from build123d import *

# Parameters (mm, degrees)
SKETCH_1_W              = 85
SKETCH_1_H              = 40
EXTRUDE_1_DEPTH         = 4
SKETCH_2_R              = 1.51
CUT_EXTRUDE_1_DEPTH     = 10
SKETCH_3_R              = 1.51
CUT_EXTRUDE_2_DEPTH     = 10
SKETCH_5_R              = 1.51
CUT_EXTRUDE_4_DEPTH     = 10
SKETCH_6_W              = 85
SKETCH_6_H              = 25
EXTRUDE_2_DEPTH         = 4
SKETCH_7_R              = 1.51
CUT_EXTRUDE_5_DEPTH     = 3
CUT_EXTRUDE_START       = -3
SKETCH_8_R              = 1.51
CUT_EXTRUDE_6_DEPTH     = 3
CUT_EXTRUDE_7_DEPTH     = 10
SKETCH_10_R             = 1.5
CUT_EXTRUDE_8_DEPTH     = 10
SKETCH_12_OUTSIDE_W     = 108.416
SKETCH_12_OUTSIDE_H     = 88.416
CUT_EXTRUDE_9_DEPTH     = 10
SKETCH_13_W             = 85
SKETCH_13_H             = 20
CUT_EXTRUDE_10_DEPTH    = 10
FILLET_2_R              = 4
MOVE_FACE_1_DEPTH       = 4
MOVE_FACE_2_OUTLINE_R   = 1.51
MOVE_FACE_2_DEPTH       = 4
MOVE_FACE_2_2_OUTLINE_R = 1.51
MOVE_FACE_2_2_DEPTH     = 4
MOVE_FACE_3_OUTLINE_R   = 1.51
MOVE_FACE_3_DEPTH       = 4
MOVE_FACE_3_2_OUTLINE_R = 1.51
MOVE_FACE_3_2_DEPTH     = 4
CUT_EXTRUDE_11_DEPTH    = 10
FILLET_3_R              = 2
CUT_EXTRUDE_12_DEPTH    = 10
FILLET_4_R              = 2


# Read off the part's stored shape, not the designer's step: 移动面1, 移动面2, 移动面3
with BuildPart() as part:
    # 草图1 → 凸台-拉伸1 (new body)
    with BuildSketch(Plane(origin=(0, 0, 0), x_dir=(0, 0, -1), z_dir=(1, 0, 0))):
        Rectangle(SKETCH_1_W, SKETCH_1_H)
    extrude(amount=EXTRUDE_1_DEPTH)

    # 草图2 → 切除-拉伸1 (cut)
    with BuildSketch(Plane.ZY):
        with Locations((-37.5, -11)):
            Circle(SKETCH_2_R)
        with Locations((37.5, -11)):
            Circle(SKETCH_2_R)
        with Locations((37.5, 11)):
            Circle(SKETCH_2_R)
        with Locations((-37.5, 11)):
            Circle(SKETCH_2_R)
    extrude(amount=-CUT_EXTRUDE_1_DEPTH, mode=Mode.SUBTRACT)

    # 草图3 → 切除-拉伸2 (cut)
    with BuildSketch(Plane.ZY):
        with Locations((-2.5, 0)):
            Circle(SKETCH_3_R)
        with Locations((-22.5, 0)):
            Circle(SKETCH_3_R)
    extrude(amount=-CUT_EXTRUDE_2_DEPTH, mode=Mode.SUBTRACT)

    # 草图5 → 切除-拉伸4 (cut)
    with BuildSketch(Plane.ZY):
        with BuildLine():
            Line((29.5, 6), (29.5, 20))
            Line((29.5, 20), (-12.5, 20))
            Line((-12.5, 20), (-12.5, 6))
            ThreePointArc((-12.5, 6), (-9.571067812, -1.071067812), (-2.5, -4))
            Line((-2.5, -4), (19.5, -4))
            ThreePointArc((19.5, -4), (26.571067812, -1.071067812), (29.5, 6))
        make_face()
        with Locations((-2.5, 0)):
            Circle(SKETCH_5_R, mode=Mode.SUBTRACT)
    extrude(amount=-CUT_EXTRUDE_4_DEPTH, mode=Mode.SUBTRACT)

    # 草图6 → 凸台-拉伸2 (add)
    with BuildSketch(Plane.ZY):
        with Locations((0, -32.5)):
            Rectangle(SKETCH_6_W, SKETCH_6_H)
    extrude(amount=-EXTRUDE_2_DEPTH)

    # 草图7 → 切除-拉伸5 (cut)
    with BuildSketch(Plane(origin=(4, 0, 0), x_dir=(0, 0, -1), z_dir=(1, 0, 0))):
        with Locations((-10, -11)):
            Circle(SKETCH_7_R)
        with Locations((10, -11)):
            Circle(SKETCH_7_R)
    extrude(amount=-CUT_EXTRUDE_5_DEPTH, mode=Mode.SUBTRACT)

    # 草图8 → 切除-拉伸6 (cut)
    with BuildSketch(Plane.ZY.offset(CUT_EXTRUDE_START)):
        with Locations(Location((-10, -11, 0), (0, 0, 180))):
            Circle(SKETCH_8_R)
        with Locations(Location((10, -11, 0), (0, 0, 180))):
            Circle(SKETCH_8_R)
    extrude(amount=CUT_EXTRUDE_6_DEPTH, mode=Mode.SUBTRACT)

    # 草图9 → 切除-拉伸7 (cut)
    with BuildSketch(Plane(origin=(4, 0, 0), x_dir=(0, 0, -1), z_dir=(1, 0, 0))):
        Polygon((26, -14), (17.872575328, -14), (-2.448990482, -14), (-16, -14), (-16, -18), (-14, -18), (24, -18), (26, -18), align=None)
    extrude(amount=-CUT_EXTRUDE_7_DEPTH, mode=Mode.SUBTRACT)

    # 草图10 → 切除-拉伸8 (cut)
    with BuildSketch(Plane(origin=(4, 0, 0), x_dir=(0, 0, -1), z_dir=(1, 0, 0))):
        with Locations((24.52, -18.02)):
            Circle(SKETCH_10_R)
        with Locations((-14.52, -18.02)):
            Circle(SKETCH_10_R)
        with Locations((-14.52, -13.98)):
            Circle(SKETCH_10_R)
        with Locations((24.52, -13.98)):
            Circle(SKETCH_10_R)
        Polygon((26.02, -13.98), (17.872575328, -13.98), (-2.448990482, -13.98), (-16.02, -13.98), (-16.02, -18.02), (-14, -18.02), (24, -18.02), (26.02, -18.02), align=None)
    extrude(amount=-CUT_EXTRUDE_8_DEPTH, mode=Mode.SUBTRACT)

    # 草图12 outside → 切除-拉伸9 (cut)
    with BuildSketch(Plane.ZY):
        with Locations((0, -12.5)):
            Rectangle(SKETCH_12_OUTSIDE_W, SKETCH_12_OUTSIDE_H)
        with BuildLine():
            Line((-12.5, 6), (-12.5, 16))
            ThreePointArc((-12.5, 16), (-13.671572875, 18.828427125), (-16.5, 20))
            Line((-16.5, 20), (-38.5, 20))
            ThreePointArc((-38.5, 20), (-41.328427125, 18.828427125), (-42.5, 16))
            Line((-42.5, 16), (-42.5, -45))
            Line((-42.5, -45), (42.5, -45))
            Line((42.5, -45), (42.5, 16))
            ThreePointArc((42.5, 16), (41.328427125, 18.828427125), (38.5, 20))
            Line((38.5, 20), (33.5, 20))
            ThreePointArc((33.5, 20), (30.671572875, 18.828427125), (29.5, 16))
            Line((29.5, 16), (29.5, 6))
            ThreePointArc((29.5, 6), (26.571067812, -1.071067812), (19.5, -4))
            Line((19.5, -4), (-2.5, -4))
            ThreePointArc((-2.5, -4), (-9.571067812, -1.071067812), (-12.5, 6))
        make_face(mode=Mode.SUBTRACT)
    extrude(amount=-CUT_EXTRUDE_9_DEPTH, mode=Mode.SUBTRACT)

    # 草图13 → 切除-拉伸10 (cut)
    with BuildSketch(Plane.ZY):
        with Locations((0, -35)):
            Rectangle(SKETCH_13_W, SKETCH_13_H)
    extrude(amount=-CUT_EXTRUDE_10_DEPTH, mode=Mode.SUBTRACT)

    # 圆角2
    fillet_2_edges = [part.edges().sort_by_distance(p)[0] for p in [
        (2, -25, 42.5),
        (2, -25, -42.5),
    ]]
    fillet(fillet_2_edges, radius=FILLET_2_R)

    # Move Face 1 outline → Move Face 1 (add)
    with BuildSketch(Plane.YZ):
        with BuildLine():
            Line((20, 38.5), (20, 45.5))
            ThreePointArc((20, 45.5), (18.828427125, 48.328427125), (16, 49.5))
            Line((16, 49.5), (-21, 49.5))
            ThreePointArc((-21, 49.5), (-23.828427125, 48.328427125), (-25, 45.5))
            Line((-25, 45.5), (-25, 38.5))
            ThreePointArc((-25, 38.5), (-23.828427125, 41.328427125), (-21, 42.5))
            Line((-21, 42.5), (16, 42.5))
            ThreePointArc((16, 42.5), (18.828427125, 41.328427125), (20, 38.5))
        make_face()
    extrude(amount=MOVE_FACE_1_DEPTH)

    # Move Face 2 outline → Move Face 2 (cut)
    with BuildSketch(Plane.YZ):
        with Locations((-21, -10)):
            Circle(MOVE_FACE_2_OUTLINE_R)
        with Locations((-21, 10)):
            Circle(MOVE_FACE_2_OUTLINE_R)
    extrude(amount=MOVE_FACE_2_DEPTH, mode=Mode.SUBTRACT)

    # Move Face 2 2 outline → Move Face 2 2 (add)
    with BuildSketch(Plane.YZ):
        with Locations((-11, -10)):
            Circle(MOVE_FACE_2_2_OUTLINE_R)
        with Locations((-11, 10)):
            Circle(MOVE_FACE_2_2_OUTLINE_R)
    extrude(amount=MOVE_FACE_2_2_DEPTH)

    # Move Face 3 outline → Move Face 3 (cut)
    with BuildSketch(Plane.YZ):
        with Locations((-6, -37.5)):
            Circle(MOVE_FACE_3_OUTLINE_R)
        with Locations((-6, 37.5)):
            Circle(MOVE_FACE_3_OUTLINE_R)
        with Locations((16, 37.5)):
            Circle(MOVE_FACE_3_OUTLINE_R)
        with Locations((16, -37.5)):
            Circle(MOVE_FACE_3_OUTLINE_R)
    extrude(amount=MOVE_FACE_3_DEPTH, mode=Mode.SUBTRACT)

    # Move Face 3 2 outline → Move Face 3 2 (add)
    with BuildSketch(Plane.YZ):
        with Locations((-11, -37.5)):
            Circle(MOVE_FACE_3_2_OUTLINE_R)
        with Locations((-11, 37.5)):
            Circle(MOVE_FACE_3_2_OUTLINE_R)
        with Locations((11, 37.5)):
            Circle(MOVE_FACE_3_2_OUTLINE_R)
        with Locations((11, -37.5)):
            Circle(MOVE_FACE_3_2_OUTLINE_R)
    extrude(amount=MOVE_FACE_3_2_DEPTH)

    # 草图14 → 切除-拉伸11 (cut)
    with BuildSketch(Plane(origin=(4, 0, 0), x_dir=(0, 0, -1), z_dir=(1, 0, 0))):
        with BuildLine():
            Line((42.5, -21), (42.5, -18))
            Line((42.5, -18), (28.5, -18))
            Line((28.5, -18), (28.5, -25))
            Line((28.5, -25), (38.5, -25))
            ThreePointArc((38.5, -25), (41.328427125, -23.828427125), (42.5, -21))
        make_face()
    extrude(amount=-CUT_EXTRUDE_11_DEPTH, mode=Mode.SUBTRACT)

    # 圆角3
    fillet_3_edges = [part.edges().sort_by_distance(p)[0] for p in [
        (2, -18, -28.5),
        (2, -25, -28.5),
        (2, -18, -42.5),
    ]]
    fillet(fillet_3_edges, radius=FILLET_3_R)

    # 草图16 → 切除-拉伸12 (cut)
    with BuildSketch(Plane.ZY):
        with BuildLine():
            Line((49.5, -18), (39.5, -18))
            Line((39.5, -18), (39.5, -25))
            Line((39.5, -25), (45.5, -25))
            ThreePointArc((45.5, -25), (48.328427125, -23.828427125), (49.5, -21))
            Line((49.5, -21), (49.5, -18))
        make_face()
    extrude(amount=-CUT_EXTRUDE_12_DEPTH, mode=Mode.SUBTRACT)

    # 圆角4
    fillet_4_edges = [part.edges().sort_by_distance(p)[0] for p in [
        (2, -18, 39.5),
        (2, -18, 49.5),
        (2, -25, 39.5),
    ]]
    fillet(fillet_4_edges, radius=FILLET_4_R)


solid = part.part
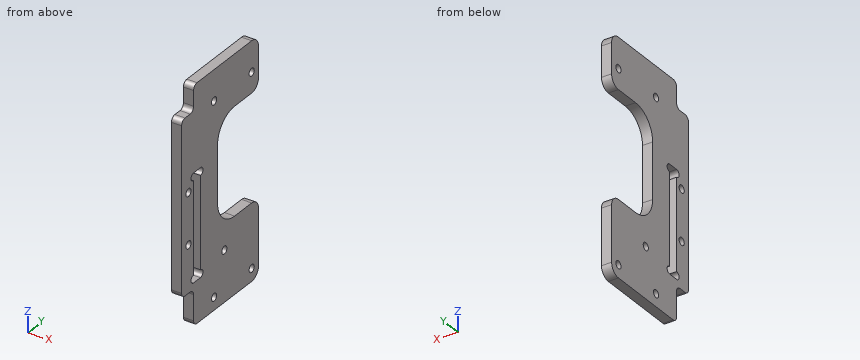
For this review, take the finished solid that the model builds, in its own axes (mm). Round coordinates to 2 decimals unless told otherwise and drop trailing zeros. Loops run counter-clockwise (first coordinate to the right, second up) from the corner with the lowest first, then second, coordinate; pieces in that order, holes last. Notation, with made-up numbers: (87.5, 26.25) - (115.5, 26.25) arc R10 cw to (115.5, 39.25) - close; hole circle Ø3 at (28, 17.5). An arc over 180 degrees is marked (long way). One line per item, written item: value. Start each with the question number.
Item 1: Take a section at C-C (y = 0). Give the boundary of the cut face in (x, z).
Item 2: Take a section at A-A (z = 14.52). Give the boundary of the cut face in (x, y), plus the area to 3 significant figures.
Item 3: For L1, parallel to Z at x = 2, y = -6; L2, parallel to Z at x = 2.5, y = 16; L3, parallel to Z at x = 0.45, y = 11, list the stretches that pass through material, from the lowest coordinate up.
Item 4: Clearance check with flat-ended pins moving along their axes: pin 1 Ø2 at (x, z) = (1.5, 10) entering from +Y; pin 2 Ø1.2 at (x, z) = (2.5, 44.5) entering from -Y. State where each tip first meets the part, or that it passes through.
Item 5: Take a section at B-B (y = 11.5). Give the boundary of the cut face in (x, z), plus the area to 3 significant figures.
Item 6: Take a section at D-D (z = -37.5). Give the boundary of the cut face in (x, y), plus the area to 3 significant figures.
Answer below:
1. outline: (0, -42.5) - (4, -42.5) - (4, -24.01) - (0, -24.01) - close; (0, -20.99) - (4, -20.99) - (4, -10.5) - (0, -10.5) - close; (0, 27.5) - (4, 27.5) - (4, 49.5) - (0, 49.5) - close
2. outline: (0, -25) - (4, -25) - (4, -19.52) - (0, -19.52) - close; (0, -12.48) - (4, -12.48) - (4, -4) - (0, -4) - close
2. area: 55.8 mm2
3. L1: z = -42.5 to -39.01, -35.99 to 35.99, 39.01 to 49.5
3. L2: z = -42.5 to -39.01, -35.99 to -12.5, 29.5 to 35.99, 39.01 to 49.5
3. L3: z = -42.5 to -12.5, 29.5 to 49.5
4. pin 1: stops at y = -4
4. pin 2: stops at y = -18
5. outline: (0, -42.5) - (4, -42.5) - (4, -12.5) - (0, -12.5) - close; (0, 29.5) - (4, 29.5) - (4, 49.5) - (0, 49.5) - close
5. area: 200 mm2
6. outline: (0, -18) - (4, -18) - (4, -7.51) - (0, -7.51) - close; (0, -4.49) - (4, -4.49) - (4, 14.49) - (0, 14.49) - close; (0, 17.51) - (4, 17.51) - (4, 20) - (0, 20) - close
6. area: 128 mm2
